Source: CAD feature listing. Evaluate the final solid. Frame: model axes, mm. Round coordinates to 2 decimals unless told otherwise and drop trailing zeros. Write each loop counter-clockwise with the first axis right and the second up, starting at its lowest first coordinate (ties: lowest second). Pieces come first, ordered by that corner, then holes. Notation, with made-up numbers: M 20.25,59.25 L 53.25,59.25 A32 ccw 53.25,96.25 Z; hole C 89.5,10.5 d7. An arc over 180 degrees is marked long. Answer in a Markdown table with one row per item.
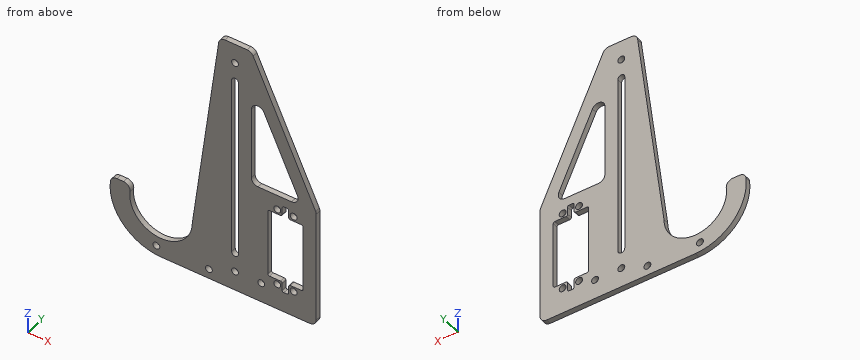
from build123d import *

# Parameters (mm, degrees)
SKETCH1_R           = 2.1
BOSS_EXTRUDE1_DEPTH = 3.2
FILLET1_R           = 4
FILLET2_R           = 1
SKETCH2_R           = 2.1
BOSS_EXTRUDE2_DEPTH = 3.2
FILLET3_R           = 4


with BuildPart() as part:
    # Sketch1 → Boss-Extrude1 (new body)
    with BuildSketch(Plane(origin=(0, 0, 0), x_dir=(1, 0, 0), z_dir=(0, 1, 0))):
        Polygon((10, 79.5), (49.480867985, 79.5), (49.480867985, 6.069914218), (10, -79.5), (-10, -79.5), (-10, 79.5), align=None)
        with Locations(Location((0, 67.5, 0), (0, 0, 270))):
            Circle(SKETCH1_R, mode=Mode.SUBTRACT)
        with Locations(Location((0, -67.5, 0), (0, 0, 270))):
            Circle(SKETCH1_R, mode=Mode.SUBTRACT)
        with Locations(Location((35.730867985, 63.569914218, 0), (0, 0, 270))):
            Circle(SKETCH1_R, mode=Mode.SUBTRACT)
        with Locations(Location((25.730867985, 63.569914218, 0), (0, 0, 270))):
            Circle(SKETCH1_R, mode=Mode.SUBTRACT)
        with Locations(Location((25.730867985, 15.069914218, 0), (0, 0, 270))):
            Circle(SKETCH1_R, mode=Mode.SUBTRACT)
        with Locations(Location((35.730867985, 15.069914218, 0), (0, 0, 270))):
            Circle(SKETCH1_R, mode=Mode.SUBTRACT)
        with Locations(Location((16, 67.5, 0), (0, 0, 270))):
            Circle(SKETCH1_R, mode=Mode.SUBTRACT)
        Polygon((19.980867985, 60.569914218), (28.730867985, 60.569914218), (28.730867985, 67.069914218), (32.730867985, 67.069914218), (32.730867985, 60.569914218), (41.480867985, 60.569914218), (41.480867985, 18.069914218), (32.730867985, 18.069914218), (32.730867985, 11.569914218), (28.730867985, 11.569914218), (28.730867985, 18.069914218), (19.980867985, 18.069914218), align=None, mode=Mode.SUBTRACT)
        with BuildLine():
            Line((-2.1, -55.5), (-2.1, 55.5))
            ThreePointArc((-2.1, 55.5), (0, 57.6), (2.1, 55.5))
            Line((2.1, 55.5), (2.1, -55.5))
            ThreePointArc((2.1, -55.5), (0, -57.6), (-2.1, -55.5))
        make_face(mode=Mode.SUBTRACT)
        Polygon((10, -60.404414159), (10, 6.069914218), (40.670408017, 6.069914218), align=None, mode=Mode.SUBTRACT)
    extrude(amount=BOSS_EXTRUDE1_DEPTH)

    # Fillet1
    fillet1_edges = [part.edges().sort_by_distance(p)[0] for p in [
        (-10, 1.6, -79.5),
        (49.480867985, 1.6, -79.5),
        (49.480867985, 1.6, -6.069914218),
        (10, 1.6, 79.5),
        (-10, 1.6, 79.5),
        (10, 1.6, 60.404414159),
        (40.670408017, 1.6, -6.069914218),
        (10, 1.6, -6.069914218),
    ]]
    fillet(fillet1_edges, radius=FILLET1_R)

    # Fillet2
    fillet2_edges = [part.edges().sort_by_distance(p)[0] for p in [
        (32.730867985, 1.6, -18.069914218),
        (41.480867985, 1.6, -18.069914218),
        (41.480867985, 1.6, -60.569914218),
        (32.730867985, 1.6, -60.569914218),
        (32.730867985, 1.6, -67.069914218),
        (28.730867985, 1.6, -67.069914218),
        (28.730867985, 1.6, -60.569914218),
        (19.980867985, 1.6, -60.569914218),
        (19.980867985, 1.6, -18.069914218),
        (28.730867985, 1.6, -18.069914218),
        (28.730867985, 1.6, -11.569914218),
        (32.730867985, 1.6, -11.569914218),
    ]]
    fillet(fillet2_edges, radius=FILLET2_R)

    # Sketch2 → Boss-Extrude2 (add)
    with BuildSketch(Plane(origin=(0, 3.2, 0), x_dir=(1, 0, 0), z_dir=(0, 1, 0))):
        with BuildLine():
            Line((-6, 79.5), (-45.05, 79.5))
            ThreePointArc((-45.05, 79.5), (-69.338886347, 67.793021998), (-75.312187627, 41.5))
            Line((-75.312187627, 41.5), (-62.786967046, 41.5))
            ThreePointArc((-62.786967046, 41.5), (-48.586472661, 67.168863777), (-26, 48.45))
            Line((-26, 48.45), (-10, -75.5))
            Line((-10, -75.5), (-10, 75.5))
            ThreePointArc((-10, 75.5), (-8.828427125, 78.328427125), (-6, 79.5))
        make_face()
        with Locations(Location((-47.914568138, 73.5, 0), (0, 0, 270))):
            Circle(SKETCH2_R, mode=Mode.SUBTRACT)
        with Locations(Location((-15.914568138, 73.5, 0), (0, 0, 270))):
            Circle(SKETCH2_R, mode=Mode.SUBTRACT)
    extrude(amount=-BOSS_EXTRUDE2_DEPTH)

    # Fillet3
    fillet3_edges = [part.edges().sort_by_distance(p)[0] for p in [
        (-62.786967046, 1.6, -41.5),
        (-75.312187627, 1.6, -41.5),
    ]]
    fillet(fillet3_edges, radius=FILLET3_R)


solid = part.part
Q1. Section C-C (z = -25). Return loops of the section in (x, y), and give its area (3 significant figures).
Solutions:
| item | result |
|---|---|
| outline | M -22.97,0 L -2.1,0 L -2.1,3.2 L -22.97,3.2 Z; M 2.1,0 L 19.98,0 L 19.98,3.2 L 2.1,3.2 Z; M 41.48,0 L 49.48,0 L 49.48,3.2 L 41.48,3.2 Z |
| area | 150 mm2 |
Q2. Section B-B (z = 67.5). Return loops of the section in (x, y), and give its area (3 significant figures).
Solutions:
| item | result |
|---|---|
| outline | M -11.03,0 L -2.1,0 L -2.1,3.2 L -11.03,3.2 Z; M 2.1,0 L 15.54,0 L 15.54,3.2 L 2.1,3.2 Z |
| area | 71.6 mm2 |
Q3. Section D-D (z = 49). Return loops of the section in (x, y).
Solutions:
| item | result |
|---|---|
| outline | M -13.42,0 L -2.1,0 L -2.1,3.2 L -13.42,3.2 Z; M 2.1,0 L 24.07,0 L 24.07,3.2 L 2.1,3.2 Z |
Q4. Material intervals for probe 1 along X at (y, z) = (1.6, -17); probe 2 along X at (y, z) = (2.4, -44.5); probe 3 along X at (y, z) = (1.45, -54.5), sorted ascending.
Solutions:
| item | result |
|---|---|
| probe 1 | x = -21.94 to -2.1, 2.1 to 24.9, 26.56 to 28.73, 32.73 to 34.9, 36.56 to 49.48 |
| probe 2 | x = -75.81 to -64.04, -25.49 to -2.1, 2.1 to 19.98, 41.48 to 49.48 |
| probe 3 | x = -75.5 to -63.11, -26.99 to -2.1, 2.1 to 19.98, 41.48 to 49.48 |
Q5. Contact query for flat-ended pins moving along their axis: pin 1 Ø1 at (x, y) = (-69.5, 1.5) entering from +Z; pin 2 Ø6.5 at (x, z) = (16, -67.5) entering from +Y; pin 3 Ø1.6 at (y, z) = (2, 16.5) entering from +X; pin 4 Ø1 at (y, z) = (2, 24) entering from +X. Output: stop coordinate, or through.
Solutions:
| item | result |
|---|---|
| pin 1 | stops at z = -41.5 |
| pin 2 | stops at y = 3.2 |
| pin 3 | stops at x = 39.44 |
| pin 4 | stops at x = 35.84 |
Q6. Section A-A (x = 0). Return loops of the section in (y, z).
Solutions:
| item | result |
|---|---|
| outline | M 0,-79.5 L 3.2,-79.5 L 3.2,-69.6 L 0,-69.6 Z; M 0,-65.4 L 3.2,-65.4 L 3.2,-57.6 L 0,-57.6 Z; M 0,57.6 L 3.2,57.6 L 3.2,65.4 L 0,65.4 Z; M 0,69.6 L 3.2,69.6 L 3.2,79.5 L 0,79.5 Z |
